from build123d import *

# Parameters (mm, degrees)
BOSS_EXTRUDE1_DEPTH = 3
SKETCH2_W           = 44
SKETCH2_H           = 44
CUT_EXTRUDE1_DEPTH  = 1.5


with BuildPart() as part:
    # Sketch1 → Boss-Extrude1 (new body)
    with BuildSketch(Plane.XY):
        with BuildLine():
            Line((-25, 24), (-25, -24))
            ThreePointArc((-25, -24), (-24.707106781, -24.707106781), (-24, -25))
            Line((-24, -25), (24, -25))
            ThreePointArc((24, -25), (24.707106781, -24.707106781), (25, -24))
            Line((25, -24), (25, 24))
            ThreePointArc((25, 24), (24.707106781, 24.707106781), (24, 25))
            Line((24, 25), (-24, 25))
            ThreePointArc((-24, 25), (-24.707106781, 24.707106781), (-25, 24))
        make_face()
    extrude(amount=-BOSS_EXTRUDE1_DEPTH)

    # Sketch2 → Cut-Extrude1 (cut)
    with BuildSketch(Plane.XY):
        Rectangle(SKETCH2_W, SKETCH2_H)
    extrude(amount=-CUT_EXTRUDE1_DEPTH, mode=Mode.SUBTRACT)

    # Sketch3 → Revolve1 (revolve)
    with BuildSketch(Plane(origin=(-10, 0, 0), x_dir=(0, 0, -1), z_dir=(1, 0, 0)), mode=Mode.PRIVATE) as revolve1_sk:
        Polygon((0, 10), (0, 11.75), (-10, 11.75), (-10, 12.25), (-7.5, 13), (1.5, 13), (1.5, 10), align=None)
    revolve(revolve1_sk.sketch.rotate(Axis((-10, 10, -1.5), (0, 0, 1)), 270), axis=Axis((-10, 10, -1.5), (0, 0, 1)))

    # Sketch4 → Revolve2 (revolve)
    with BuildSketch(Plane(origin=(10, 0, 0), x_dir=(0, 0, -1), z_dir=(1, 0, 0)), mode=Mode.PRIVATE) as revolve2_sk:
        Polygon((0, 10), (0, 11.75), (-10, 11.75), (-10, 12.25), (-7.5, 13), (1.5, 13), (1.5, 10), align=None)
    revolve(revolve2_sk.sketch.rotate(Axis((10, 10, -1.5), (0, 0, 1)), 270), axis=Axis((10, 10, -1.5), (0, 0, 1)))

    # Sketch5 → Revolve3 (revolve)
    with BuildSketch(Plane(origin=(10, 0, 0), x_dir=(0, 0, -1), z_dir=(1, 0, 0)), mode=Mode.PRIVATE) as revolve3_sk:
        Polygon((0, -10), (0, -8.25), (-10, -8.25), (-10, -7.75), (-7.5, -7), (1.5, -7), (1.5, -10), align=None)
    revolve(revolve3_sk.sketch.rotate(Axis((10, -10, -1.5), (0, 0, 1)), 270), axis=Axis((10, -10, -1.5), (0, 0, 1)))

    # Sketch6 → Revolve4 (revolve)
    with BuildSketch(Plane(origin=(-10, 0, 0), x_dir=(0, 0, -1), z_dir=(1, 0, 0)), mode=Mode.PRIVATE) as revolve4_sk:
        Polygon((0, -10), (0, -8.25), (-10, -8.25), (-10, -7.75), (-7.5, -7), (1.5, -7), (1.5, -10), align=None)
    revolve(revolve4_sk.sketch.rotate(Axis((-10, -10, -1.5), (0, 0, 1)), 270), axis=Axis((-10, -10, -1.5), (0, 0, 1)))


solid = part.part
Model file for the job. Use its own axes, mm. A direction names the side the tool comes from. Give positions to 0.01 mm unless a question says otherwise; leave off trailing zeros. Loops run counter-clockwise (first coordinate to the right, second up) from the corner with the lowest first, then second, coordinate; pieces in that order, holes last. Notation, with made-up numbers: (74.25, 56.5) - (129.25, 56.5) arc R11 cw to (129.25, 69.5) - close; hole circle Ø4 at (-33, 74). An arc over 180 degrees is marked (long way). Use one line per item in the form item = value.
(1) Cut at B-B (x = -10). Give the cut face in (y, z).
Determined:
outline = (-25, -3) - (25, -3) - (25, 0) - (22, 0) - (22, -1.5) - (13, -1.5) - (13, 7.5) - (12.25, 10) - (11.75, 10) - (11.75, 0) - (8.25, 0) - (8.25, 10) - (7.75, 10) - (7, 7.5) - (7, -1.5) - (-7, -1.5) - (-7, 7.5) - (-7.75, 10) - (-8.25, 10) - (-8.25, 0) - (-11.75, 0) - (-11.75, 10) - (-12.25, 10) - (-13, 7.5) - (-13, -1.5) - (-22, -1.5) - (-22, 0) - (-25, 0) - close
(2) Cut at A-A (z = 1.5). Give the cut face in (x, y), then the cut area to 3 significant figures.
Determined:
outline = circle Ø6 at (-10, -10); circle Ø6 at (-10, 10); circle Ø6 at (10, -10); circle Ø6 at (10, 10); hole circle Ø3.5 at (-10, -10); hole circle Ø3.5 at (-10, 10); hole circle Ø3.5 at (10, -10); hole circle Ø3.5 at (10, 10)
area = 74.6 mm^2
(3) Cut at C-C (y = 0). Give the cut face in (x, z), then the cut area to 3 significant figures.
Determined:
outline = (-25, -3) - (25, -3) - (25, 0) - (22, 0) - (22, -1.5) - (-22, -1.5) - (-22, 0) - (-25, 0) - close
area = 84.0 mm^2
(4) Drill centre lines: L1, parallel to Y at x = -10, z = 5.75; L2, parallel to Y at x = 12, z = -0.25; L3, parallel to X at y = 1, z = -0.75. Where is each one in solid material? Low to high.
Determined:
L1 = -13 to -11.75, -8.25 to -7, 7 to 8.25, 11.75 to 13
L2 = -25 to -22, -12.24 to -7.76, 7.76 to 12.24, 22 to 25
L3 = -25 to -22, 22 to 25
(5) Pull direction Y, two halves, no side cores. Call faces 1 (the face through (0, 25, -1)), 2 (the face through (0, -25, -1)), 3 (the face through (-10, -10, 0)): pulls with the +Y half, pulls with the -Y half, needs draft (parallel to the pull), parting line crosses it, or undercut.
Determined:
face_1 = pulls with the +Y half
face_2 = pulls with the -Y half
face_3 = undercut
(6) 3-axis set-ups, long thin cutter, end or side, ignore diameter. For faces 4 (the face through (10, -12, 10)), 5 (the face through (0, -22, -1)): which of +Z, -Z, +X, -X, +Y, -Y reach the whole face in a straight line?
Determined:
face_4 = +Z, +X, -X, +Y, -Y
face_5 = +Z
(7) Drop flat-ended pins along their axis: P1, Ø1.5, axis at y = -6.5, z = 1.5, coming from the +X side; P2, Ø2, axis at y = 11, z = 8.5, coming from the +X side; P3, Ø1.5, axis at y = -6, z = 7.5, coming from the -X side; P4, Ø1, axis at x = -10, y = -11, coming from the +Z side. Give the stop position or say it passes through.
Determined:
P1 = 11.2
P2 = 12.92
P3 = through
P4 = 0
